Part model, mm, in its own coordinate system. A direction names the side the tool comes from. Round coordinates to 2 decimals unless told otherwise and drop trailing zeros. Loops run counter-clockwise (first coordinate to the right, second up) from the corner with the lowest first, then second, coordinate; pieces in that order, holes last.
(1) Probe probe 1 along Z at (x, y) = (0, -29); probe 2 along Y at (x, z) = (-10, 17); probe 3 along Z at (x, y) = (0, 14). List the from-to ranges inside material, lowest first.
(2) Mould opens along Y. For faces 3 (the face through (28.728, 3.104, -9.047)), 4 (the face through (0, -36.336, 6)), 5 (the face through (-2.619, 3.944, -19.947)) say: +Y half, -Y half, draft (parallel to the pull), parting line (faces both ways), or undercut.
(3) Cut at D-D on y = -3. List the corners of the cut face in (x, z).
(4) Cut at C-C on z = 13.5. List the corners of the cut face in (x, y), then the cut area to 3 significant figures.
(5) Flat gauge pins, fed straight in: pin 1 (10 mm diameter, centred on y = 13.5, z = 23.5, fed in from +X); pin 2 (8 mm diameter, centred on x = -21.5, y = 31, fed in from +Z); pin 3 (1.5 mm diameter, centred on x = -12, y = -26, fed in from -Z). Where does each tip first touch, or does it go through?
(6) Cut at B-B on x = 0. List the corners of the cut face in (y, z), then the cut area to 3 significant figures.
(7) Cut at A-A on z = 0. List the corners of the cut face in (x, y), then the cut area to 3 significant figures.
(8) Tool access for faces 1 (the face through (4.88, 33.8, -1.54)), 2 (the face through (-4, -16.336, 4)): list every direction of +Z, -Z, +X, -X, +Y, -Y with a clear straight run to the whole face (end or side of a thin tool).
from build123d import *


with BuildPart() as part:
    # Croquis6 → Revolución2 (revolve)
    with BuildSketch(Plane.XY):
        Polygon((5.118334973, 43.663840535), (30.118334973, 43.663840535), (30.118334973, -36.336159465), (5.118334973, -36.336159465), (5.118334973, -16.336159465), (20.118334973, -16.336159465), (20.118334973, 23.663840535), (5.118334973, 23.663840535), align=None)
    revolve(axis=Axis((0, 0, 0), (0, 1, 0)))


solid = part.part
Final values:
1. probe 1: z = -30.12 to -5.12, 5.12 to 30.12
1. probe 2: y = -36.34 to -16.34, 23.66 to 43.66
1. probe 3: z = -30.12 to -20.12, 20.12 to 30.12
2. face 3: draft
2. face 4: -Y half
2. face 5: undercut
3. outline: circle Ø60.24 at (0, 0); hole circle Ø40.24 at (0, 0)
4. outline: (-26.92, -36.34) - (26.92, -36.34) - (26.92, 43.66) - (-26.92, 43.66) - close; hole (-14.92, -16.34) - (14.92, -16.34) - (14.92, 23.66) - (-14.92, 23.66) - close
4. area: 3,110 mm2
5. pin 1: stops at x = 23.77
5. pin 2: stops at z = 24.51
5. pin 3: stops at z = -27.94
6. outline: (-36.34, -30.12) - (43.66, -30.12) - (43.66, -5.12) - (23.66, -5.12) - (23.66, -20.12) - (-16.34, -20.12) - (-16.34, -5.12) - (-36.34, -5.12) - close; (-36.34, 5.12) - (-16.34, 5.12) - (-16.34, 20.12) - (23.66, 20.12) - (23.66, 5.12) - (43.66, 5.12) - (43.66, 30.12) - (-36.34, 30.12) - close
6. area: 2,800 mm2
7. outline: (-30.12, -36.34) - (-5.12, -36.34) - (-5.12, -16.34) - (-20.12, -16.34) - (-20.12, 23.66) - (-5.12, 23.66) - (-5.12, 43.66) - (-30.12, 43.66) - close; (5.12, -36.34) - (30.12, -36.34) - (30.12, 43.66) - (5.12, 43.66) - (5.12, 23.66) - (20.12, 23.66) - (20.12, -16.34) - (5.12, -16.34) - close
7. area: 2,800 mm2
8. face 1: +Y, -Y
8. face 2: none
